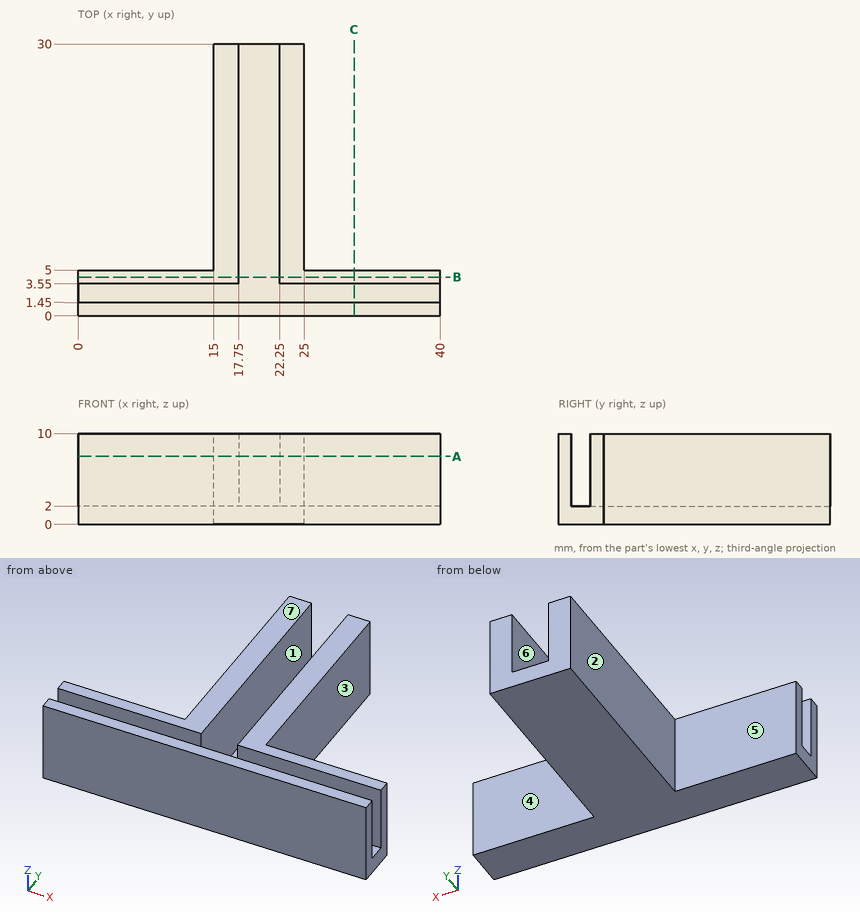
Drawing for the job (mm, zero at the part's lowest x, y, z). A direction names the side the tool comes from. Give positions to 0.01 mm unless a question says otherwise; leave off trailing zeros. Loops run counter-clockwise (first coordinate to the right, second up) from the corner with the lowest first, then second, coordinate; pieces in that order, holes last.
1) Probe line 1 along Y through (x, z) = (35.5, 8); line 2 along Y through (x, z) = (17.5, 9); line 3 along X through (y, z) = (24.5, 6.75). List the from-to ranges inside material, lowest first.
Values follow:
line 1: y = 0 to 1.45, 3.55 to 5
line 2: y = 0 to 1.45, 3.55 to 30
line 3: x = 15 to 17.75, 22.25 to 25
2) 3-axis set-ups, long thin cutter, end or side, ignore diameter. For the marked faces 5, 6 and 7: which of +Z, -Z, +X, -X, +Y, -Y reach the whole face in a straight line?
Values follow:
face 5: +Z, -Z, -X, +Y
face 6: +Z, +Y
face 7: +Z, +X, -X, +Y, -Y
3) Two-plate mould, pull along X, no slides. Class the marked faces 1, 2, 3 and 4: released by +X, released by -X, zero draft, split by the parting line, or undercut.
Values follow:
face 1: undercut
face 2: released by -X
face 3: released by +X
face 4: zero draft
4) Band-saw the part on C-C on x = 30.5. List the corners of the cut face in (y, z), then the cut area to 3 significant figures.
Values follow:
outline: (0, 0) - (5, 0) - (5, 10) - (3.55, 10) - (3.55, 2) - (1.45, 2) - (1.45, 10) - (0, 10) - close
area: 33.2 mm2
5) Band-saw the part on A-A on z = 7.5. List the corners of the cut face in (x, y).
Values follow:
outline: (0, 0) - (40, 0) - (40, 1.45) - (0, 1.45) - close; (0, 3.55) - (17.75, 3.55) - (17.75, 30) - (15, 30) - (15, 5) - (0, 5) - close; (22.25, 3.55) - (40, 3.55) - (40, 5) - (25, 5) - (25, 30) - (22.25, 30) - close
6) Band-saw the part on B-B on y = 4.25. List the corners of the cut face in (x, z), then the cut area to 3 significant figures.
Values follow:
outline: (0, 0) - (40, 0) - (40, 10) - (22.25, 10) - (22.25, 2) - (17.75, 2) - (17.75, 10) - (0, 10) - close
area: 364 mm2
7) Drop flat-ended pins along their axis: P1, Ø6, axis at y = 20.5, z = 1, coming from the -X side; P2, Ø8.5, axis at x = 11, y = 9, coming from the +Z side; P3, Ø1.5, axis at y = 12.5, z = 4.5, coming from the +X side; P4, Ø1, axis at x = 12.5, z = 4, coming from the +Y side. Give the stop position or say it passes through.
Values follow:
P1: stops at x = 15
P2: stops at z = 10
P3: stops at x = 25
P4: stops at y = 5
